Input: part model. Units: mm. Frame: model coordinates. A direction names the side the tool comes from. Round coordinates to 2 decimals unless told otherwise and drop trailing zeros. Write each loop counter-clockwise with the first axis right and the second up, starting at its lowest first coordinate (ties: lowest second). Pieces come first, ordered by that corner, then holes. Notation, with made-up numbers: M 13,-19.75 L 60,-19.75 A3 ccw 60,-14.75 Z; hole C 53,-1.5 d11. An arc over 180 degrees is marked long. Write each question's results on one line, items separated by ' | '. Start each with the question number.
```python
from build123d import *

# Parameters (mm, degrees)
F0_R     = 50.1
F0_R_2   = 4.5
F1_DEPTH = 3
F2_R     = 4.5
F3_DEPTH = 25
F4_R     = 2.99999
F5_R     = 5


# Not quite as in the source:
# - a fillet or chamfer is up to 0.001 mm smaller than in the source, because OpenCascade refuses the exact size


with BuildPart() as f1:
    # F0 (on Front) → F1 (new body)
    with BuildSketch(Plane.XZ):
        Circle(F0_R)
        Circle(F0_R_2, mode=Mode.SUBTRACT)
    extrude(amount=F1_DEPTH)

    # F2 (on face) → F3 (join)
    with BuildSketch(Plane.XZ.offset(3)):
        Polygon((9.4680966624, -8.46690492), (2.598506421, 12.4330646951), (-12.0666030834, -3.9661597751), align=None)
        Circle(F2_R, mode=Mode.SUBTRACT)
    extrude(amount=F3_DEPTH)

    # F4 (radius 3 in the source; OpenCascade refuses exactly that, so slightly less here)
    f4_edges = [f1.edges().sort_by_distance(p)[0] for p in [
        (-50.1, 0, 0),
    ]]
    fillet(f4_edges, radius=F4_R)

    # F5
    f5_edges = [f1.edges().sort_by_distance(p)[0] for p in [
        (2.598506, -15.5, 12.433065),
        (-12.066603, -15.5, -3.96616),
        (9.468097, -15.5, -8.466905),
    ]]
    fillet(f5_edges, radius=F5_R)


solid = f1.part
```
1. Access query for faces 4 (the face through (-4.71, -15.32, 4.26)), 5 (the face through (-7.293, -15.675, -2.474)), 6 (the face through (6.044, -15.325, 1.952)). Directions: +Z, -Z, +X, -X, +Y, -Y. A direction counts if a zero-diameter tool reaches every point of the face in a straight line with its end or side. Return the directions, or none.
2. Line query: L1, parallel to Y at x = -19, z = 22; L2, parallel to Z at x = 0, y = -18.5; L3, parallel to X at y = -10.5, z = 3.5. Output: solid intervals per line, ascending. Write a range as from..to.
3. Draft query along Z for faces 1 (the face through (-1, -3, -10)), 2 (the face through (-0.59, -13.8, 4.46)), 3 (the face through (1.647, -15.675, 7.523)). Return one class per face: +Z half, -Z half, draft (parallel to the pull), parting line (faces both ways), or undercut.
4. Cut plane A-A on y = -16.5. Output: boundary loops of the cut face in (x, z).
5. Contact query for flat-ended pins moving along their axis: P1, Ø10, axis at x = -26.5, z = -3, coming from the -Y side; P2, Ø1, axis at y = -5, z = 22.5, coming from the +X side; P3, Ø10, axis at y = -22.5, z = -4.5, coming from the +X side. Output: stop coordinate, or through.
Answers follow:
1) face 4: +Z, -X, -Y | face 5: -X, -Y | face 6: +Z, +X, -Y
2) L1: y = -3..0 | L2: z = -6.49..-4.5, 4.5..7.61 | L3: x = -5.39..-2.83, 2.83..5.53
3) face 1: draft | face 2: undercut | face 3: +Z half
4) outline: M -6.29,2.49 A5 ccw -3.59,-5.74 L 0.99,-6.7 A5 ccw 6.76,-0.24 L 5.3,4.21 A5 ccw -3.17,5.98 Z; hole C 0,0 d9
5) P1: stops at y = -3 | P2: passes through | P3: stops at x = 7.01
